The model under review builds one solid part; all positions refer to its coordinate system, in mm. A direction names the side the tool comes from. Coordinates: 2 decimals unless noted, no trailing zeros. Order: outer loops, then holes, each group sorted by start corner. A loop starts at its lowest first (then second) coordinate and runs counter-clockwise, first axis right, second up. Notation, with made-up numbers: (-17, 70) - (16, 70) arc R9 cw to (16, 81) - close; hole circle Ø1 at (29.25, 7.25). An arc over 180 degrees is marked (long way). Answer in a Markdown table with one row per item.
```python
from build123d import *

# Parameters (mm, degrees)
SKETCH_1_R               = 50
EXTRUDE_1_DEPTH          = 42
SKETCH_2_R               = 47.45
CUT_EXTRUDE_1_DEPTH      = 9
SKETCH_3_R               = 43
CUT_EXTRUDE_2_DEPTH      = 5
SKETCH_4_R               = 1.7
CUT_EXTRUDE_3_DEPTH      = 49
SKETCH_5_R               = 50
SKETCH_5_R_2             = 32
SKETCH_5_R_3             = 1.7
CUT_EXTRUDE_4_DEPTH      = 20
FILLET_1_R               = 2
FILLET_2_R               = 2
SKETCH_6_R               = 1.7
CUT_EXTRUDE_5_DEPTH      = 83.24354078
CUT_EXTRUDE_5_DEPTH_BACK = 83.24354078
SKETCH_7_R               = 3
CUT_EXTRUDE_6_DEPTH      = 17.5
SKETCH_8_R               = 3
CUT_EXTRUDE_7_DEPTH      = 8
SKETCH_9_R               = 2.1
CUT_EXTRUDE_8_DEPTH      = 5
SKETCH_10_R              = 3
CUT_EXTRUDE_9_DEPTH      = 2.5
SKETCH_11_R              = 50
SKETCH_11_R_2            = 32
CUT_EXTRUDE_10_DEPTH     = 83.24354078
FILLET_3_R               = 3


with BuildPart() as part:
    # 草图1 → 凸台-拉伸1 (new body)
    with BuildSketch(Plane.XY):
        with Locations(Location((0, 0, 0), (0, 0, 180))):
            Circle(SKETCH_1_R)
    extrude(amount=EXTRUDE_1_DEPTH)

    # 草图2 → 切除-拉伸1 (cut)
    with BuildSketch(Plane(origin=(0, 0, 0), x_dir=(-1, 0, 0), z_dir=(0, 0, -1))):
        Circle(SKETCH_2_R)
    extrude(amount=-CUT_EXTRUDE_1_DEPTH, mode=Mode.SUBTRACT)

    # 草图3 → 切除-拉伸2 (cut)
    with BuildSketch(Plane(origin=(0, 0, 9), x_dir=(-1, 0, 0), z_dir=(0, 0, -1))):
        Circle(SKETCH_3_R)
    extrude(amount=-CUT_EXTRUDE_2_DEPTH, mode=Mode.SUBTRACT)

    # 草图4 → 切除-拉伸3 (cut)
    with BuildSketch(Plane(origin=(0, 0, 14), x_dir=(-1, 0, 0), z_dir=(0, 0, -1))):
        with Locations((0, -18)):
            Circle(SKETCH_4_R)
        with Locations((-15.588457268, -9)):
            Circle(SKETCH_4_R)
        with Locations((-15.588457268, 9)):
            Circle(SKETCH_4_R)
        with Locations((0, 18)):
            Circle(SKETCH_4_R)
        with Locations((15.588457268, 9)):
            Circle(SKETCH_4_R)
        with Locations((15.588457268, -9)):
            Circle(SKETCH_4_R)
    extrude(amount=-CUT_EXTRUDE_3_DEPTH, mode=Mode.SUBTRACT)

    # 草图5 → 切除-拉伸4 (cut)
    with BuildSketch(Plane.XY.offset(42)):
        with Locations(Location((0, 0, 0), (0, 0, 180))):
            Circle(SKETCH_5_R)
        Circle(SKETCH_5_R_2, mode=Mode.SUBTRACT)
        with BuildLine():
            Line((10, 0), (23, 0))
            ThreePointArc((23, 0), (22.18603902, -6.06462469), (19.801767598, -11.7))
            Line((19.801767598, -11.7), (24.333310502, -11.7))
            ThreePointArc((24.333310502, -11.7), (0, 27), (-24.333310502, -11.7))
            Line((-24.333310502, -11.7), (-19.801767598, -11.7))
            ThreePointArc((-19.801767598, -11.7), (-22.18603902, -6.06462469), (-23, 0))
            Line((-23, 0), (-10, 0))
            Line((-10, 0), (-10, -8))
            Line((-10, -8), (10, -8))
            Line((10, -8), (10, 0))
        make_face()
        with Locations(Location((-15.588457268, 9, 0), (0, 0, 180))):
            Circle(SKETCH_5_R_3, mode=Mode.SUBTRACT)
        with Locations(Location((0, 18, 0), (0, 0, 180))):
            Circle(SKETCH_5_R_3, mode=Mode.SUBTRACT)
        with Locations(Location((15.588457268, 9, 0), (0, 0, 180))):
            Circle(SKETCH_5_R_3, mode=Mode.SUBTRACT)
    extrude(amount=-CUT_EXTRUDE_4_DEPTH, mode=Mode.SUBTRACT)

    # 圆角1
    fillet_1_edges = [part.edges().sort_by_distance(p)[0] for p in [
        (50, 0, 22),
    ]]
    fillet(fillet_1_edges, radius=FILLET_1_R)

    # 圆角2
    fillet_2_edges = [part.edges().sort_by_distance(p)[0] for p in [
        (-32, 0, 22),
    ]]
    fillet(fillet_2_edges, radius=FILLET_2_R)

    # 草图6 → 切除-拉伸5 (cut, two sides)
    with BuildSketch(Plane(origin=(0, 0, 0), x_dir=(1, 0, 0), z_dir=(0, 1, 0))) as cut_extrude_5_sk:
        with Locations(Location((-15, -32.2, 0), (0, 0, 270))):
            Circle(SKETCH_6_R)
        with Locations(Location((15, -32.2, 0), (0, 0, 270))):
            Circle(SKETCH_6_R)
    extrude(amount=CUT_EXTRUDE_5_DEPTH, mode=Mode.SUBTRACT)
    extrude(cut_extrude_5_sk.sketch, amount=-CUT_EXTRUDE_5_DEPTH_BACK, mode=Mode.SUBTRACT)

    # 草图7 → 切除-拉伸6 (cut)
    with BuildSketch(Plane.XY.offset(42)):
        with Locations((-15.588457268, -9)):
            Circle(SKETCH_7_R)
        with Locations((0, -18)):
            Circle(SKETCH_7_R)
        with Locations((15.588457268, -9)):
            Circle(SKETCH_7_R)
    extrude(amount=-CUT_EXTRUDE_6_DEPTH, mode=Mode.SUBTRACT)

    # 草图8 → 切除-拉伸7 (cut)
    with BuildSketch(Plane(origin=(0, -23, 0), x_dir=(1, 0, 0), z_dir=(0, 1, 0))):
        with Locations(Location((-15, -32.2, 0), (0, 0, 270))):
            Circle(SKETCH_8_R)
        with Locations(Location((15, -32.2, 0), (0, 0, 270))):
            Circle(SKETCH_8_R)
    extrude(amount=-CUT_EXTRUDE_7_DEPTH, mode=Mode.SUBTRACT)

    # 草图9 → 切除-拉伸8 (cut, symmetric)
    with BuildSketch(Plane(origin=(0, 25, 0), x_dir=(1, 0, 0), z_dir=(0, 1, 0))):
        with Locations(Location((-15, -32.2, 0), (0, 0, 270))):
            Circle(SKETCH_9_R)
        with Locations(Location((15, -32.2, 0), (0, 0, 270))):
            Circle(SKETCH_9_R)
    extrude(amount=CUT_EXTRUDE_8_DEPTH, both=True, mode=Mode.SUBTRACT)

    # 草图10 → 切除-拉伸9 (cut)
    with BuildSketch(Plane.XY.offset(22)):
        with Locations((-15.588457268, 9)):
            Circle(SKETCH_10_R)
        with Locations((0, 18)):
            Circle(SKETCH_10_R)
        with Locations((15.588457268, 9)):
            Circle(SKETCH_10_R)
    extrude(amount=-CUT_EXTRUDE_9_DEPTH, mode=Mode.SUBTRACT)

    # 草图11 → 切除-拉伸10 (cut, through all)
    with BuildSketch(Plane.XY.offset(42)):
        Circle(SKETCH_11_R)
        Circle(SKETCH_11_R_2, mode=Mode.SUBTRACT)
    extrude(amount=-CUT_EXTRUDE_10_DEPTH, mode=Mode.SUBTRACT)

    # 圆角3
    fillet_3_edges = [part.edges().sort_by_distance(p)[0] for p in [
        (-32, 0, 14),
    ]]
    fillet(fillet_3_edges, radius=FILLET_3_R)


solid = part.part
```
Item 1: We need section A-A, the plane x = 0. Write out the cut boundary in (y, z), then the cut area to 3 significant figures.
Check values:
| item | result |
|---|---|
| outline | (-32, 17) arc R3 ccw to (-29, 14) - (-19.7, 14) - (-19.7, 24.5) - (-21, 24.5) - (-21, 42) - (-32, 42) - close; (-16.3, 14) - (16.3, 14) - (16.3, 19.5) - (15, 19.5) - (15, 22) - (-8, 22) - (-8, 42) - (-15, 42) - (-15, 24.5) - (-16.3, 24.5) - close; (19.7, 14) - (29, 14) arc R3 ccw to (32, 17) - (32, 42) - (27, 42) - (27, 22) - (21, 22) - (21, 19.5) - (19.7, 19.5) - close |
| area | 914 mm^2 |
Item 2: We need section B-B, the plane z = 37. Write out the cut boundary in (x, y).
Check values:
| item | result |
|---|---|
| outline | circle Ø64 at (0, 0); hole (-24.33, -11.7) - (-19.8, -11.7) arc R23 cw to (-23, 0) - (-10, 0) - (-10, -8) - (10, -8) - (10, 0) - (23, 0) arc R23 cw to (19.8, -11.7) - (24.33, -11.7) arc R27 ccw (long way) to start; hole circle Ø6 at (-15.59, -9); hole circle Ø6 at (0, -18); hole circle Ø6 at (15.59, -9) |
Item 3: Mouldability with a two-part tool opening along X and no side actions: class faces 4 (the face through (12.07, -25.55, 31.55)), 5 (the face through (0, 0, 14)) as +X half, -X half, draft (parallel to the pull), parting line (faces both ways), or undercut.
Check values:
| item | result |
|---|---|
| face 4 | undercut |
| face 5 | draft |
Item 4: We need section C-C, the plane z = 16. Write out the cut boundary in (x, y).
Check values:
| item | result |
|---|---|
| outline | circle Ø63.66 at (0, 0); hole circle Ø3.4 at (-15.59, -9); hole circle Ø3.4 at (-15.59, 9); hole circle Ø3.4 at (0, -18); hole circle Ø3.4 at (0, 18); hole circle Ø3.4 at (15.59, -9); hole circle Ø3.4 at (15.59, 9) |
Item 5: We need section D-D, the plane y = -18. State how many separate pieces and enclosed holes the cut face has, then the cut area to 3 significant figures.
Check values:
| item | result |
|---|---|
| separate pieces | 2 |
| enclosed holes | 2 |
| area | 1,320 mm^2 |
Item 6: To check wall thickness, follow line 1 (Y direction, x = -20.5, z = 25.25); line 2 (Y direction, x = 2, z = 39); line 3 (Z direction, x = 10, y = 1). State the ranges of each line that lie inside material, in increasing order. Write a range as from..to.
Check values:
| item | result |
|---|---|
| line 1 | -24.57..-11.7, -10.43..0, 17.57..24.57 |
| line 2 | -31.94..-20.24, -15.76..-8, 26.93..31.94 |
| line 3 | 14..22 |
Item 7: Tool access review of faces 1 (the face through (17.082, 25.148, 31.927)), 2 (the face through (13, -23, 32)), 3 (the face through (-14, 8, 19.5)): name each direction out of +Z, -Z, +X, -X, +Y, -Y from which nothing blocks a thin tool from reaching the whole face with its end or side.
Check values:
| item | result |
|---|---|
| face 1 | +Y |
| face 2 | -Y |
| face 3 | +Z |
Item 8: Clearance check with flat-ended pins moving along their axes: pin 1 Ø1.8 at (x, y) = (16, -8) entering from +Z; pin 2 Ø6 at (x, z) = (2, 30) entering from +Y; pin 3 Ø9.5 at (x, z) = (15, 32.2) entering from +Y; pin 4 Ø3 at (x, z) = (-15, 32.2) entering from +Y. State where each tip first meets the part, or that it passes through.
Check values:
| item | result |
|---|---|
| pin 1 | z = 24.5 |
| pin 2 | y = 32 |
| pin 3 | y = 30.31 |
| pin 4 | through |
